Verification items for this drawing (mm, ordinates from the low corner). Round coordinates to 2 decimals unless told otherwise and drop trailing zeros. Loops run counter-clockwise (first coordinate to the right, second up) from the corner with the lowest first, then second, coordinate; pieces in that order, holes last. Notation, with made-up numbers: (79.25, -9.5) - (134.25, -9.5) arc R24 ccw to (134.25, 8.5) - close; hole circle Ø1 at (43.25, -4.75). An arc over 180 degrees is marked (long way). Write item = value, one per line.
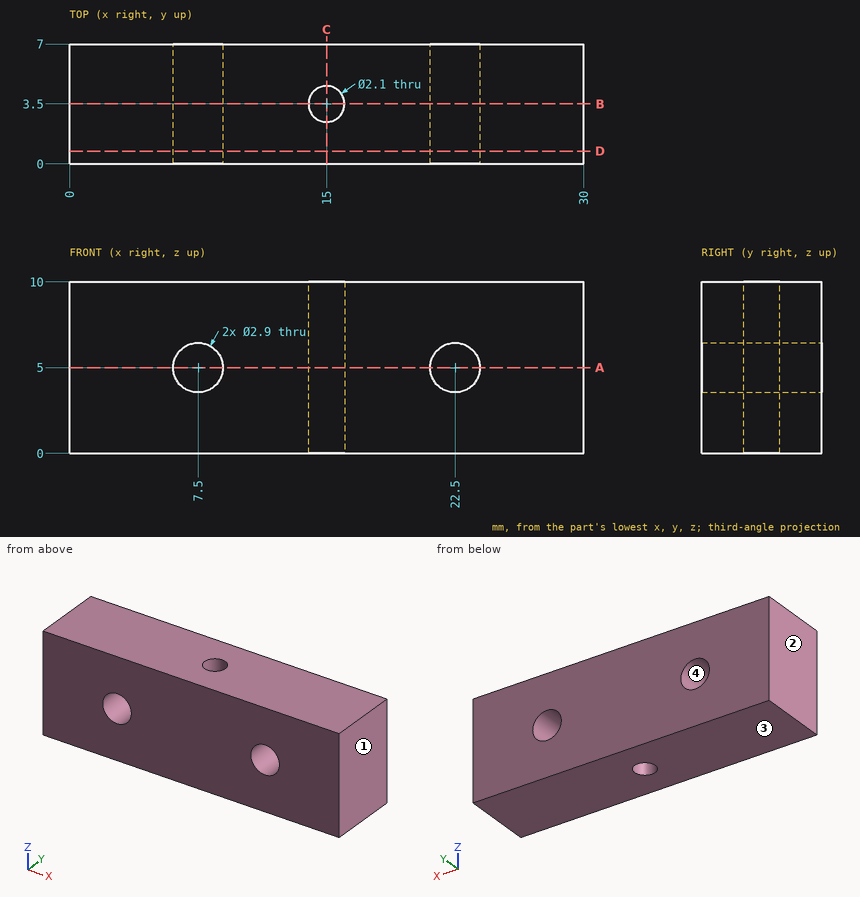
(1) Mould release check, pull along X, two halves, no side actions. Record for the marked faces 1, 2, 3 and 4: pulls with the +X half, pulls with the -X half, needs draft (parallel to the pull), parting line crosses it, or undercut.
Answers follow:
face_1 = pulls with the +X half
face_2 = pulls with the -X half
face_3 = needs draft
face_4 = undercut
(2) Section check C-C (x = 15). Enter the section's corners in (y, z), then the cut area to 3 significant figures.
Answers follow:
outline = (0, 0) - (2.45, 0) - (2.45, 10) - (0, 10) - close; (4.55, 0) - (7, 0) - (7, 10) - (4.55, 10) - close
area = 49.0 mm²
(3) Section check A-A (z = 5). Enter the section's corners in (x, y), then the cut area to 3 significant figures.
Answers follow:
outline = (0, 0) - (6.05, 0) - (6.05, 7) - (0, 7) - close; (8.95, 0) - (21.05, 0) - (21.05, 7) - (8.95, 7) - close; (23.95, 0) - (30, 0) - (30, 7) - (23.95, 7) - close; hole circle Ø2.1 at (15, 3.5)
area = 166 mm²
(4) Section check D-D (y = 0.75). Enter the section's corners in (x, z), then the cut area to 3 significant figures.
Answers follow:
outline = (0, 0) - (30, 0) - (30, 10) - (0, 10) - close; hole circle Ø2.9 at (7.5, 5); hole circle Ø2.9 at (22.5, 5)
area = 287 mm²
(5) Scan lines: L1, parallel to X at y = 1, z = 5; L2, parallel to X at y = 4, z = 5; L3, parallel to Z at x = 7.5, y = 4.5. Record each from-to range of solid material in increasing order. Write a range as [from, to].
Answers follow:
L1 = [0, 6.05], [8.95, 21.05], [23.95, 30]
L2 = [0, 6.05], [8.95, 14.08], [15.92, 21.05], [23.95, 30]
L3 = [0, 3.55], [6.45, 10]
(6) Gauge pin test, flat end, axial feed: pin 1 (1.7 mm diameter, centred on x = 22.5, z = 5, fed in from -Y). Record the tip position at first contact, or that the pin passes through.
Answers follow:
pin_1 = through
(7) Section check B-B (y = 3.5). Enter the section's corners in (x, z).
Answers follow:
outline = (0, 0) - (13.95, 0) - (13.95, 10) - (0, 10) - close; (16.05, 0) - (30, 0) - (30, 10) - (16.05, 10) - close; hole circle Ø2.9 at (7.5, 5); hole circle Ø2.9 at (22.5, 5)
